Geometry check sheet. Reference: the model listing, model coordinates, mm. Face numbers are marked on the shaded views. A direction names the side the tool comes from. Coordinates: 2 decimals unless noted, no trailing zeros. Write each loop counter-clockwise with the first axis right and the second up, starting at its lowest first coordinate (ties: lowest second). Pieces come first, ordered by that corner, then holes. Notation, with made-up numbers: (6, 78) -> (57, 78) arc R20 cw to (57, 98) -> close; hole circle Ø11 at (56, 77.5). An arc over 180 degrees is marked (long way). One line per question, with ' | ' between items.
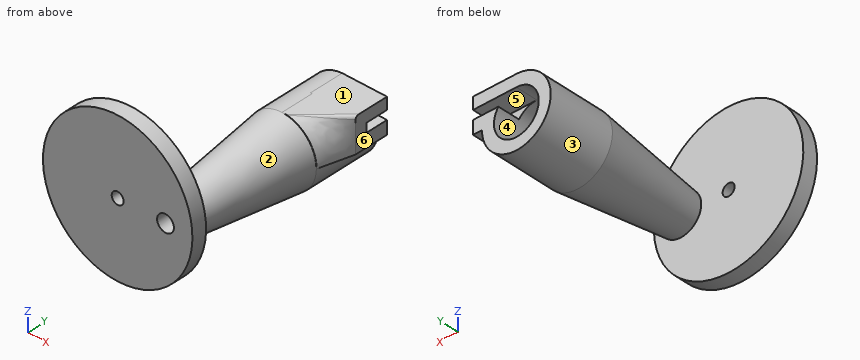
```python
from build123d import *

# Parameters (mm, degrees)
BOSS_EXTRUDE2_DEPTH = 15
SKETCH9_W           = 3
SKETCH9_H           = 7.5
CUT_EXTRUDE2_DEPTH  = 14.5
SKETCH10_R          = 7.5
CUT_EXTRUDE3_DEPTH  = 19
FILLET2_R           = 1
BOSS_EXTRUDE3_START = -5
SKETCH13_R          = 25
SKETCH13_R_2        = 2.815
SKETCH13_R_3        = 2
BOSS_EXTRUDE3_DEPTH = 5


with BuildPart() as part:
    # Sketch1 → Revolve1 (revolve)
    with BuildSketch(Plane.XY, mode=Mode.PRIVATE) as revolve1_sk:
        Polygon((2.815, 0), (7.5, 37.747281127), (7.5, 60), (11.5, 60), (11.5, 37.5), (6.845691272, 0), (8, 0), (8, -5), (2.815, -4.99976246), align=None)
    revolve(revolve1_sk.sketch.rotate(Axis((0, 0, 0), (0, 1, 0)), 90), axis=Axis((0, 0, 0), (0, 1, 0)))

    # Sketch8 → Boss-Extrude2 (add)
    with BuildSketch(Plane(origin=(14.5, 0, 0), x_dir=(0, 0, -1), z_dir=(1, 0, 0))):
        Polygon((-7.5, 60), (-11.5, 60), (-11.5, 48.5), (0, 48.5), (0, 60), (-4.5, 60), (-4.5, 52.5), (-7.5, 52.5), align=None)
    extrude(amount=-BOSS_EXTRUDE2_DEPTH)

    # Sketch9 → Cut-Extrude2 (cut)
    with BuildSketch(Plane(origin=(14.5, 0, 0), x_dir=(0, 0, -1), z_dir=(1, 0, 0))):
        with Locations((-6, 56.25)):
            Rectangle(SKETCH9_W, SKETCH9_H)
    extrude(amount=-CUT_EXTRUDE2_DEPTH, mode=Mode.SUBTRACT)

    # Sketch10 → Cut-Extrude3 (cut)
    with BuildSketch(Plane(origin=(0, 60, 0), x_dir=(1, 0, 0), z_dir=(0, 1, 0))):
        with Locations(Location((0, 0, 0), (0, 0, 90))):
            Circle(SKETCH10_R)
    extrude(amount=-CUT_EXTRUDE3_DEPTH, mode=Mode.SUBTRACT)

    # Sketch11 for Loft4 → Loft4 section 0
    with BuildSketch(Plane.XZ.offset(-48.5)):
        with BuildLine():
            Line((0, 11.5), (14.5, 11.5))
            Line((14.5, 11.5), (14.5, 0))
            Line((14.5, 0), (11.5, 0))
            # circular arc as an exact rational Bezier (weights 1, cos(half-angle), 1)
            Bezier((11.5, 0), (11.5, 11.5), (0, 11.5), weights=[1, 0.707106781, 1])
        make_face()
    # Sketch12 for Loft4 → Loft4 section 1
    with BuildSketch(Plane(origin=(0, 37.5, 0), x_dir=(1, 0, 0), z_dir=(0, 1, 0))):
        with BuildLine():
            Line((0, -11.5), (1.519868415, -11.5))
            Bezier((1.519868415, -11.5), (11.6, -10.167784903), (11.6, 0), weights=[1, 0.752005033, 1])
            Line((11.6, 0), (11.5, 0))
            Bezier((11.5, 0), (11.5, -11.5), (0, -11.5), weights=[1, 0.707106781, 1])
        make_face()
    loft()

    # Fillet2
    fillet2_edges = [part.edges().sort_by_distance(p)[0] for p in [
        (8.009934208, 43, 11.5),
    ]]
    fillet(fillet2_edges, radius=FILLET2_R)

    # Sketch13 → Boss-Extrude3 (add)
    with BuildSketch(Plane.XZ.offset(5).offset(BOSS_EXTRUDE3_START)):
        with Locations(Location((-16, 0, 0), (0, 0, 270))):
            Circle(SKETCH13_R)
        with Locations(Location((0, 0, 0), (0, 0, 270))):
            Circle(SKETCH13_R_2, mode=Mode.SUBTRACT)
        with Locations(Location((-16, 0, 0), (0, 0, 270))):
            Circle(SKETCH13_R_3, mode=Mode.SUBTRACT)
    extrude(amount=BOSS_EXTRUDE3_DEPTH)


solid = part.part
```
(1) Tool access check on the marked faces 1, 2 and 3. Record the directions out of +Z, -Z, +X, -X, +Y, -Y that give a thin tool (end or side, any length) a straight path to the whole face; none if there is none.
Answers below:
face 1: +Z, +X, -X, +Y | face 2: none | face 3: +Y
(2) Cross-section at C-C (x = -27.5). Record the cut outline in (y, z).
Answers below:
outline: (-5, -22.2) -> (0, -22.2) -> (0, 22.2) -> (-5, 22.2) -> close
(3) Cross-section at A-A (x = -16). Record the cut outline in (y, z), plus the area to 3 significant figures.
Answers below:
outline: (-5, -25) -> (0, -25) -> (0, -2) -> (-5, -2) -> close; (-5, 2) -> (0, 2) -> (0, 25) -> (-5, 25) -> close | area: 230 mm²
(4) Depth check by flat-ended pin: P1, Ø25, axis at x = -26, z = -12, coming from the +Y side; P2, Ø2.5, axis at x = -16, z = 0, coming from the +Y side; P3, Ø2, axis at x = 3.5, y = 47.5, coming from the -Z side (3 decimals); P4, Ø7.5, axis at x = 8, y = 46.5, coming from the +Z side. Enter the tip coordinate at first touch or a pass-through.
Answers below:
P1: stops at y = 0 | P2: passes through | P3: stops at z = -11.225 | P4: stops at z = 11.5
(5) Cross-section at B-B (z = -20). Record the cut outline in (x, y).
Answers below:
outline: (-31, -5) -> (-1, -5) -> (-1, 0) -> (-31, 0) -> close
(6) Material ranges on line 1 (X direction, y = -3.1, z = 0) (3 decimals); line 2 (Y direction, x = -8, z = 17); line 3 (Z direction, x = 0, y = -2) (3 decimals), recorded low to high.
Answers below:
line 1: x = -41 to -18, -14 to -2.815, 2.815 to 9 | line 2: y = -5 to 0 | line 3: z = -19.209 to -2.815, 2.815 to 19.209
(7) Draft check along X on the marked faces 4, 5 and 6. Enter one of: pulls with the +X half, pulls with the -X half, needs draft (parallel to the pull), parting line crosses it, or undercut.
Answers below:
face 4: undercut | face 5: needs draft | face 6: pulls with the +X half
